Build history of the part. All positions in model axes, mm. A direction names the side the tool comes from. Round coordinates to 2 decimals unless told otherwise and drop trailing zeros. Loops run counter-clockwise (first coordinate to the right, second up) from the corner with the lowest first, then second, coordinate; pieces in that order, holes last.
from build123d import *

# Parameters (mm, degrees)
SKETCH_W        = 40
SKETCH_H        = 40
SKETCH_R        = 5.05
PAD_DEPTH       = 10
SKETCH001_R     = 1.3
POCKET_DEPTH    = 10.001
SKETCH002_R     = 2.6
POCKET001_DEPTH = 8.7
SKETCH005_R     = 1.5
POCKET003_DEPTH = 10.001
POCKET004_DEPTH = 6
SKETCH006_R     = 18.5
POCKET005_DEPTH = 6
SKETCH007_R     = 17.5
POCKET006_DEPTH = 2.5
FILLET_R        = 1


with BuildPart() as part:
    # Sketch → Pad (new body)
    with BuildSketch(Plane.XY):
        Rectangle(SKETCH_W, SKETCH_H)
        Circle(SKETCH_R, mode=Mode.SUBTRACT)
    extrude(amount=PAD_DEPTH)

    # Sketch001 (on Face7 of Pad) → Pocket (cut, through all)
    with BuildSketch(Plane.XY.offset(10)):
        with Locations((8, 0)):
            Circle(SKETCH001_R)
        with Locations((-8, 0)):
            Circle(SKETCH001_R)
    extrude(amount=-POCKET_DEPTH, mode=Mode.SUBTRACT)

    # Sketch002 (on Face5 of Pocket) → Pocket001 (cut)
    with BuildSketch(Plane.XY.offset(10)):
        with Locations((-8, 0)):
            Circle(SKETCH002_R)
        with Locations((8, 0)):
            Circle(SKETCH002_R)
    extrude(amount=-POCKET001_DEPTH, mode=Mode.SUBTRACT)

    # Sketch005 (on Face5 of Pocket001) → Pocket003 (cut, through all)
    with BuildSketch(Plane.XY.offset(10)):
        with Locations((-16, 16)):
            Circle(SKETCH005_R)
        with Locations((16, 16)):
            Circle(SKETCH005_R)
        with Locations((-16, -16)):
            Circle(SKETCH005_R)
        with Locations((16, -16)):
            Circle(SKETCH005_R)
    extrude(amount=-POCKET003_DEPTH, mode=Mode.SUBTRACT)

    # Sketch004 (on Face5 of Pocket003) → Pocket004 (cut)
    with BuildSketch(Plane.XY.offset(10)):
        with BuildLine():
            Line((13.434683, 15.312625), (15.312625, 13.434683))
            Line((15.312625, 13.434683), (15.35345, 13.393859))
            ThreePointArc((15.35345, 13.393859), (16.802339, 13.00563), (17.862999, 14.06629))
            Line((17.877942, 14.122058), (17.862999, 14.06629))
            Line((17.877942, 14.122058), (18.565317, 16.687375))
            Line((18.565317, 16.687375), (18.58026, 16.743142))
            ThreePointArc((18.58026, 16.743142), (18.192031, 18.192031), (16.743142, 18.58026))
            Line((16.687375, 18.565317), (16.743142, 18.58026))
            Line((16.687375, 18.565317), (14.122058, 17.877942))
            Line((14.122058, 17.877942), (14.06629, 17.862999))
            ThreePointArc((14.06629, 17.862999), (13.00563, 16.802339), (13.393859, 15.35345))
            Line((13.434683, 15.312625), (13.393859, 15.35345))
        make_face()
        with BuildLine():
            Line((14.122058, -17.877942), (16.687375, -18.565317))
            Line((16.687375, -18.565317), (16.743142, -18.58026))
            ThreePointArc((16.743142, -18.58026), (18.192031, -18.192031), (18.58026, -16.743142))
            Line((18.565317, -16.687375), (18.58026, -16.743142))
            Line((18.565317, -16.687375), (17.877942, -14.122058))
            Line((17.877942, -14.122058), (17.862999, -14.06629))
            ThreePointArc((17.862999, -14.06629), (16.802339, -13.00563), (15.35345, -13.393859))
            Line((15.312625, -13.434683), (15.35345, -13.393859))
            Line((15.312625, -13.434683), (13.434683, -15.312625))
            Line((13.434683, -15.312625), (13.393859, -15.35345))
            ThreePointArc((13.393859, -15.35345), (13.00563, -16.802339), (14.06629, -17.862999))
            Line((14.122058, -17.877942), (14.06629, -17.862999))
        make_face()
        with BuildLine():
            Line((-14.122058, 17.877942), (-16.687375, 18.565317))
            Line((-16.687375, 18.565317), (-16.743142, 18.58026))
            ThreePointArc((-16.743142, 18.58026), (-18.192031, 18.192031), (-18.58026, 16.743142))
            Line((-18.565317, 16.687375), (-18.58026, 16.743142))
            Line((-18.565317, 16.687375), (-17.877942, 14.122058))
            Line((-17.877942, 14.122058), (-17.862999, 14.06629))
            ThreePointArc((-17.862999, 14.06629), (-16.802339, 13.00563), (-15.35345, 13.393859))
            Line((-15.312625, 13.434683), (-15.35345, 13.393859))
            Line((-15.312625, 13.434683), (-13.434683, 15.312625))
            Line((-13.434683, 15.312625), (-13.393859, 15.35345))
            ThreePointArc((-13.393859, 15.35345), (-13.00563, 16.802339), (-14.06629, 17.862999))
            Line((-14.122058, 17.877942), (-14.06629, 17.862999))
        make_face()
        with BuildLine():
            Line((-13.434683, -15.312625), (-15.312625, -13.434683))
            Line((-15.312625, -13.434683), (-15.35345, -13.393859))
            ThreePointArc((-15.35345, -13.393859), (-16.802339, -13.00563), (-17.862999, -14.06629))
            Line((-17.877942, -14.122058), (-17.862999, -14.06629))
            Line((-17.877942, -14.122058), (-18.565317, -16.687375))
            Line((-18.565317, -16.687375), (-18.58026, -16.743142))
            ThreePointArc((-18.58026, -16.743142), (-18.192031, -18.192031), (-16.743142, -18.58026))
            Line((-16.687375, -18.565317), (-16.743142, -18.58026))
            Line((-16.687375, -18.565317), (-14.122058, -17.877942))
            Line((-14.122058, -17.877942), (-14.06629, -17.862999))
            ThreePointArc((-14.06629, -17.862999), (-13.00563, -16.802339), (-13.393859, -15.35345))
            Line((-13.434683, -15.312625), (-13.393859, -15.35345))
        make_face()
    extrude(amount=-POCKET004_DEPTH, mode=Mode.SUBTRACT)

    # Sketch006 (on Face5 of Pocket004) → Pocket005 (cut)
    with BuildSketch(Plane.XY.offset(10)):
        Circle(SKETCH006_R)
    extrude(amount=-POCKET005_DEPTH, mode=Mode.SUBTRACT)

    # Sketch007 (on Face67 of Pocket005) → Pocket006 (cut)
    with BuildSketch(Plane.XY.offset(4)):
        Circle(SKETCH007_R)
    extrude(amount=-POCKET006_DEPTH, mode=Mode.SUBTRACT)

    # Fillet
    fillet_edges = [part.edges().sort_by_distance(p)[0] for p in [
        (20, -20, 5),
        (-20, -20, 5),
        (-20, 20, 5),
        (20, 20, 5),
    ]]
    fillet(fillet_edges, radius=FILLET_R)


solid = part.part
(1) Slice it at B-B on y = 0. Count the separate pieces of the cut face and the enclosed holes in it, plus the area to 3 significant figures.
Responses:
separate pieces: 4
enclosed holes: 0
area: 66.5 mm2
(2) Pull direction Y, two halves, no side cores. Call faces 1 (the face through (18.207, 18.176, 7.042)), 2 (the face through (-5, 5, 0)), 3 (the face through (0, 20, 5)): +Y half, -Y half, draft (parallel to the pull), parting line (faces both ways), or undercut.
Responses:
face 1: undercut
face 2: draft
face 3: +Y half
(3) Slice it at D-D on y = -7.5. List the corners of the cut face in (x, z), plus the area to 3 significant figures.
Responses:
outline: (-20, 0) - (20, 0) - (20, 10) - (16.91, 10) - (16.91, 4) - (15.81, 4) - (15.81, 1.5) - (-15.81, 1.5) - (-15.81, 4) - (-16.91, 4) - (-16.91, 10) - (-20, 10) - close
area: 118 mm2
(4) Which spindle directions (+Z, -Z, +X, -X, +Y, -Y) get a long thin tool onto all of the face, cutting with end or side? Do faces 4 (the face through (-19.715, 19.699, 5.07)), 5 (the face through (-16, -14, 4)). Say none if no direction does.
Responses:
face 4: +Z, -Z, -X, +Y
face 5: +Z
(5) Probe line 1 (X direction, y = -15, z = 7); line 2 (Y direction, x = 8, z = 0.45); line 3 (Y direction, x = -8, z = 6.5). List the from-to ranges inside material, lowest first.
Responses:
line 1: x = -20 to -18.11, -13.75 to -10.83, 10.83 to 13.75, 18.11 to 20
line 2: y = -20 to -1.3, 1.3 to 20
line 3: y = -20 to -16.68, 16.68 to 20
(6) Slice it at A-A on x = 0. List the corners of the cut face in (y, z), plus the area to 4 significant figures.
Responses:
outline: (-20, 0) - (-5.05, 0) - (-5.05, 1.5) - (-17.5, 1.5) - (-17.5, 4) - (-18.5, 4) - (-18.5, 10) - (-20, 10) - close; (5.05, 0) - (20, 0) - (20, 10) - (18.5, 10) - (18.5, 4) - (17.5, 4) - (17.5, 1.5) - (5.05, 1.5) - close
area: 75.35 mm2
(7) Pin check, flat tips, straight feed: P1, Ø5.5, axis at x = -7.5, y = -1, coming from the +Z side; P2, Ø1.7, axis at x = 14.5, y = 16.5, coming from the +Z side. Stop position of each tip, or through.
Responses:
P1: stops at z = 1.5
P2: stops at z = 4
